```python
from build123d import *

# Parameters (mm, degrees)
SKETCH006_W     = 108.5
SKETCH006_H     = 65
PAD003_DEPTH    = 23
SKETCH007_W     = 52
SKETCH007_H     = 62
SKETCH007_H_2   = 53
POCKET003_DEPTH = 21.5
POCKET004_DEPTH = 280.109926
FILLET003_R     = 1
FILLET004_R     = 0.5


with BuildPart() as part:
    # Sketch006 → Pad003 (new body)
    with BuildSketch(Plane.XY):
        Rectangle(SKETCH006_W, SKETCH006_H)
    extrude(amount=PAD003_DEPTH)

    # Sketch007 (on DatumPlane) → Pocket003 (cut)
    with BuildSketch(Plane.XY.offset(23)):
        with Locations((-26.75, 0)):
            Rectangle(SKETCH007_W, SKETCH007_H)
        with Locations((26.75, 4.5)):
            Rectangle(SKETCH007_W, SKETCH007_H_2)
    extrude(amount=-POCKET003_DEPTH, mode=Mode.SUBTRACT)

    # Sketch008 (on DatumPlane) → Pocket004 (cut, through all)
    with BuildSketch(Plane(origin=(-26.75, 0, 23), x_dir=(1, 0, 0), z_dir=(0, 0, 1))):
        with BuildLine():
            Line((10, 0), (10, 40))
            Line((10, 40), (-10, 40))
            Line((-10, 40), (-10, 0))
            ThreePointArc((-10, 0), (0, -10.840906), (10, 0))
        make_face()
    pocket004 = extrude(amount=-POCKET004_DEPTH, mode=Mode.SUBTRACT)

    # Mirrored002: Pocket004 across YZ
    add(pocket004.mirror(Plane.YZ), mode=Mode.SUBTRACT)

    # Fillet003
    fillet003_edges = [part.edges().sort_by_distance(p)[0] for p in [
        (-45.5, 32.5, 0),
        (-36.75, 16.25, 0),
        (-26.75, -10.840906, 0),
        (-16.75, 16.25, 0),
        (0, 32.5, 0),
        (16.75, 16.25, 0),
        (26.75, -10.840906, 0),
        (36.75, 16.25, 0),
        (45.5, 32.5, 0),
        (54.25, 0, 0),
        (0, -32.5, 0),
        (-54.25, 0, 0),
    ]]
    fillet(fillet003_edges, radius=FILLET003_R)

    # Fillet004
    fillet004_edges = [part.edges().sort_by_distance(p)[0] for p in [
        (-45.5, 32.5, 23),
        (-36.75, 31.75, 23),
        (-44.75, 31, 23),
        (-52.75, 0, 23),
        (-26.75, -31, 23),
        (-0.75, 0, 23),
        (-8.75, 31, 23),
        (-16.75, 31.75, 23),
        (0, 32.5, 23),
        (16.75, 31.75, 23),
        (8.75, 31, 23),
        (0.75, 4.5, 23),
        (26.75, -22, 23),
        (52.75, 4.5, 23),
        (44.75, 31, 23),
        (36.75, 31.75, 23),
        (45.5, 32.5, 23),
        (54.25, 0, 23),
        (0, -32.5, 23),
        (-54.25, 0, 23),
    ]]
    fillet(fillet004_edges, radius=FILLET004_R)


with BuildPart() as part_1:
    # Body002 placement: moved
    add(part.part.moved(Location((-41, 113, 14))))


solid = part_1.part
```
Verification items for the finished model (mm, model axes). A direction names the side the tool comes from. Coordinates: 2 decimals unless noted, no trailing zeros. Order: outer loops, then holes, each group sorted by start corner. A loop starts at its lowest first (then second) coordinate and runs counter-clockwise, first axis right, second up. Notation, with made-up numbers: (30, 76) -> (84, 76) arc R15 cw to (84, 101) -> close; hole circle Ø1 at (-30, -22). An arc over 180 degrees is marked (long way). Answer as CSV lines item,"result". Start each with the question number.
1) Cross-section at A-A, the plane y = 125. Give the number of separate pieces and of enclosed holes in the cut face, then the cut area to 3 significant figures.
2) Gauge pin test, flat ends, axial feed: pin 1 Ø10.5 at (x, z) = (-11.5, 30) entering from +Y; pin 2 Ø10 at (x, y) = (-62, 135) entering from -Z; pin 3 Ø2 at (x, y) = (-46, 130) entering from +Z. Record the tip position at first contact, or that the pin passes through.
3) Cross-section at D-D, the plane x = -67.75. Record the boundary of the cut face in (y, z), then the cut area to 3 significant figures.
4) Cross-section at B-B, the plane z = 33.75. Record the boundary of the cut face in (x, y).
5) Material ranges on L1, parallel to X at y = 136.5, z = 34; L2, parallel to Y at x = -53.5, z = 36.25; L3, parallel to Y at x = -2, z = 17.5, recorded low to high. Write a range as [from, to].
6) Release check for a two-part mould opening along X. For faces 3 (the face through (13.25, 113, 26)), 4 (the face through (-40.25, 117, 26)), 5 (the face through (4, 145.5, 26)) record: released by +X, released by -X, zero draft, split by the parting line, or undercut.
7) Set-up check for faces 1 (the face through (-42, 80.5, 26)), 2 (the face through (-15, 91, 26)): record each of +Z, -Z, +X, -X, +Y, -Y from which the full face is reachable in a straight line by a thin tool's end or side.
8) Cross-section at C-C, the plane y = 95. Record the boundary of the cut face in (x, z).
Conclusion:
1,separate pieces,"3"
1,enclosed holes,"0"
1,area,"198 mm²"
2,pin 1,"stops at y = 91"
2,pin 2,"stops at z = 14.03"
2,pin 3,"stops at z = 15.5"
3,outline,"(80.5, 15) arc R1 ccw to (81.5, 14) -> (101.16, 14) arc R1 ccw to (102.16, 15) -> (102.16, 15.5) -> (82, 15.5) -> (82, 36.5) arc R0.5 ccw to (81.5, 37) -> (81, 37) arc R0.5 ccw to (80.5, 36.5) -> close"
3,area,"64.2 mm²"
4,outline,"(-95.25, 80.5) -> (13.25, 80.5) -> (13.25, 145.5) -> (-4.25, 145.5) -> (-4.25, 144) -> (11.75, 144) -> (11.75, 91) -> (-40.25, 91) -> (-40.25, 144) -> (-24.25, 144) -> (-24.25, 145.5) -> (-57.75, 145.5) -> (-57.75, 144) -> (-41.75, 144) -> (-41.75, 82) -> (-93.75, 82) -> (-93.75, 144) -> (-77.75, 144) -> (-77.75, 145.5) -> (-95.25, 145.5) -> close"
5,L1,"x = [-95.25, -93.75], [-41.75, -40.25], [11.75, 13.25]"
5,L2,"y = [80.5, 82], [144, 145.5]"
5,L3,"y = [80.5, 91], [144, 145.5]"
6,face 3,"released by +X"
6,face 4,"undercut"
6,face 5,"zero draft"
7,face 1,"+Z, -Z, +X, -X, -Y"
7,face 2,"+Z"
8,outline,"(-95.25, 15) arc R1 ccw to (-94.25, 14) -> (12.25, 14) arc R1 ccw to (13.25, 15) -> (13.25, 36.5) arc R0.5 ccw to (12.75, 37) -> (12.25, 37) arc R0.5 ccw to (11.75, 36.5) -> (11.75, 15.5) -> (-40.25, 15.5) -> (-40.25, 36.5) arc R0.5 ccw to (-40.75, 37) -> (-41.25, 37) arc R0.5 ccw to (-41.75, 36.5) -> (-41.75, 15.5) -> (-93.75, 15.5) -> (-93.75, 36.5) arc R0.5 ccw to (-94.25, 37) -> (-94.75, 37) arc R0.5 ccw to (-95.25, 36.5) -> close"
